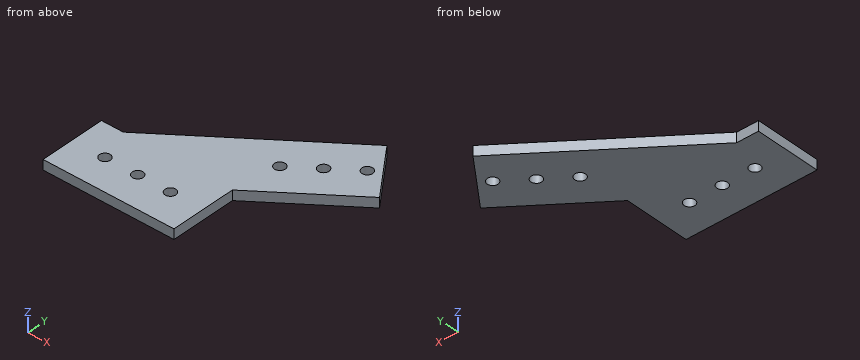
```python
from build123d import *

# Parameters (mm, degrees)
SKETCH_1_R      = 1.65
EXTRUDE_1_DEPTH = 3


with BuildPart() as part:
    # 草图1 → 凸台-拉伸1 (new body)
    with BuildSketch(Plane.XY):
        Polygon((-18.830697363, -8.06225338), (-25.497363461, -8.06225338), (-25.497363461, -28.06225338), (14.502631424, -28.06225338), (14.502631424, -8.06225338), (41.408851068, 12.117415653), (29.408849432, 28.117414426), align=None)
        with Locations((-5.497363461, -18.06225338)):
            Circle(SKETCH_1_R, mode=Mode.SUBTRACT)
        with Locations((4.502636539, -18.06225338)):
            Circle(SKETCH_1_R, mode=Mode.SUBTRACT)
        with Locations((-15.497363461, -18.06225338)):
            Circle(SKETCH_1_R, mode=Mode.SUBTRACT)
        with Locations((16.502629992, 5.937746824)):
            Circle(SKETCH_1_R, mode=Mode.SUBTRACT)
        with Locations((24.502629378, 11.937747642)):
            Circle(SKETCH_1_R, mode=Mode.SUBTRACT)
        with Locations((32.502628764, 17.937748461)):
            Circle(SKETCH_1_R, mode=Mode.SUBTRACT)
    extrude(amount=EXTRUDE_1_DEPTH)


solid = part.part
```
CAD build for the part. Positions are in the model's coordinates, mm. Round coordinates to 2 decimals unless told otherwise and drop trailing zeros. Order: outer loops, then holes, each group sorted by start corner. A loop starts at its lowest first (then second) coordinate and runs counter-clockwise, first axis right, second up.
Q1. Wall check: L1, parallel to X at y = 17, z = 2.2; L2, parallel to Y at x = 6, z = 2.5; L3, parallel to Y at x = 32.5, z = 0.2. Give the ranges that are in metal, low to high.
Q2. Slice it at D-D (x = 33). Write the cut outline in (y, z), and give its area (3 significant figures).
Q3. Slice it at A-A (x = 4.5). Write the cut outline in (y, z), and give its area (3 significant figures).
Q4. Drop flat-ended pins along their axis: pin 1 (3 mm diameter, centred on x = 32.5, y = 17.94, fed in from +Z); pin 2 (1 mm diameter, centred on y = -21.5, z = 0.5, fed in from +X); pin 3 (1.5 mm diameter, centred on x = -6, z = 0.5, fed in from +Y). Give the stop position or say it passes through.
Q5. Slice it at B-B (z = 2.5). Write the cut outline in (x, y), and give its area (3 significant figures).
Q6. Slice it at C-C (y = -15.5). Write the cut outline in (x, z), and give its area (3 significant figures).
Results below:
1. L1: x = 14.59 to 31.15, 33.86 to 37.75
1. L2: y = -28.06 to -18.76, -17.37 to 10.56
1. L3: y = 5.44 to 16.29, 19.59 to 24
2. outline: (5.81, 0) - (16.36, 0) - (16.36, 3) - (5.81, 3) - close; (19.51, 0) - (23.33, 0) - (23.33, 3) - (19.51, 3) - close
2. area: 43.1 mm2
3. outline: (-28.06, 0) - (-19.71, 0) - (-19.71, 3) - (-28.06, 3) - close; (-16.41, 0) - (9.44, 0) - (9.44, 3) - (-16.41, 3) - close
3. area: 103 mm2
4. pin 1: passes through
4. pin 2: stops at x = 14.5
4. pin 3: stops at y = 2.12
5. outline: (-25.5, -28.06) - (14.5, -28.06) - (14.5, -8.06) - (41.41, 12.12) - (29.41, 28.12) - (-18.83, -8.06) - (-25.5, -8.06) - close; hole circle Ø3.3 at (-15.5, -18.06); hole circle Ø3.3 at (-5.5, -18.06); hole circle Ø3.3 at (4.5, -18.06); hole circle Ø3.3 at (16.5, 5.94); hole circle Ø3.3 at (24.5, 11.94); hole circle Ø3.3 at (32.5, 17.94)
5. area: 1,690 mm2
6. outline: (-25.5, 0) - (14.5, 0) - (14.5, 3) - (-25.5, 3) - close
6. area: 120 mm2
